Can you work these out from the drawing? Everything is in mm from the part's minimum corner. Give positions to 0.01 mm unless a question says otherwise; leave off trailing zeros. Write each loop counter-clockwise with the first axis right and the second up, starting at its lowest first coordinate (ties: lowest second). Pieces come first, ordered by that corner, then holes. Notation, with made-up numbers: (72, 1.5) - (87, 1.5) arc R23 ccw to (87, 38.5) - close; hole circle Ø1 at (-17.5, 23). An arc over 180 degrees is marked (long way). Return JSON: item names as keys, results as strings. Group by question number.
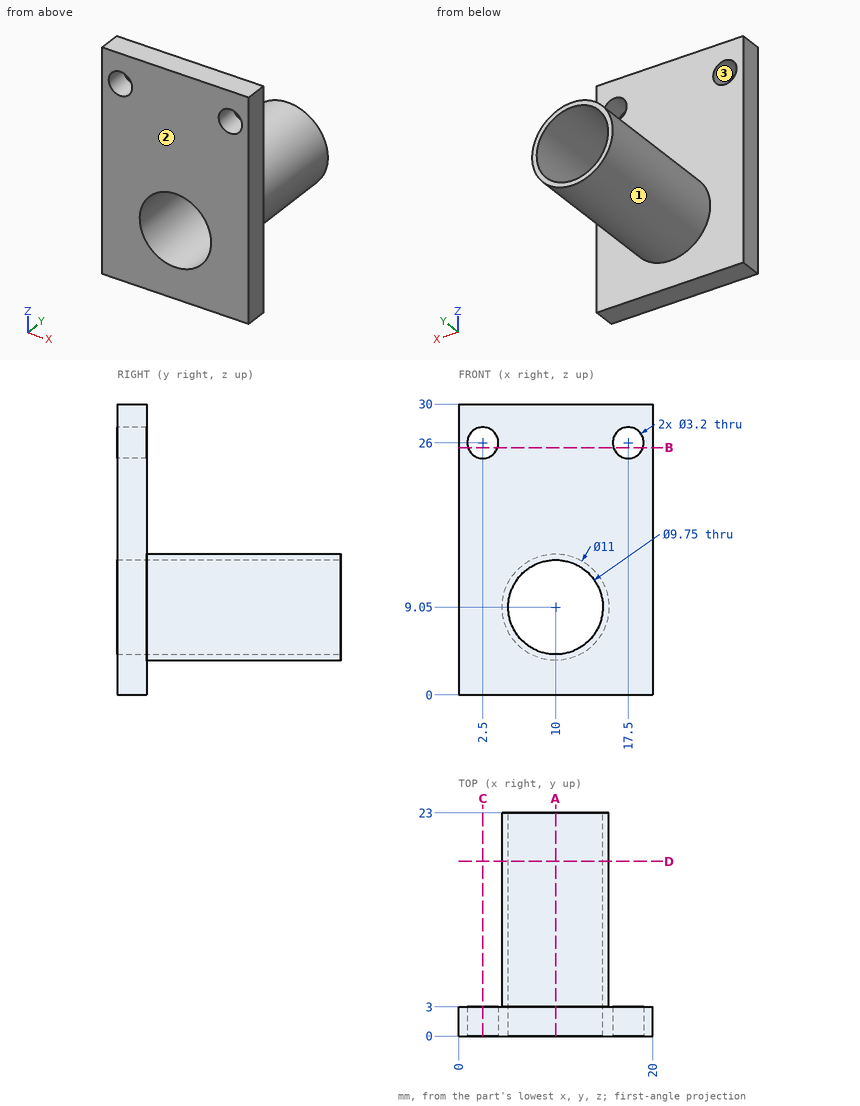
1) Will these pins go through, and if not, where does the flat tip stop? pin 1 Ø8 at (y, z) = (20, 20.5) entering from -X; pin 2 Ø6 at (x, y) = (11.5, 12.5) entering from +Z; pin 3 Ø4 at (x, z) = (11.5, 19.5) entering from +Y; pin 4 Ø2 at (y, z) = (5.5, 4.5) entering from +X.
2) Imagine slicing it at A-A, the plane x = 10. Write out the boundary of the cut face in (y, z) (3 decimals).
3) Imagine slicing it at B-B, the plane z = 25.5. Write out the boundary of the cut face in (x, y), and give its area (3 significant figures).
4) Imagine slicing it at D-D, the plane y = 18. Write out the boundary of the cut face in (x, z) (3 decimals).
5) Imagine slicing it at C-C, the plane x = 2.5. Write out the boundary of the cut face in (y, z).
6) We'd pull the mould along X, two halves only. Please class the marked faces 1, 2 and 3: pulls with the +X half, pulls with the -X half, needs draft (parallel to the pull), parting line crosses it, or undercut.
7) I need wall thicknesses on line 1 along X through (y, z) = (0.7, 26); line 2 along X through (y, z) = (5.75, 9.05) (3 decimals); line 3 along Y through (x, z) = (5, 1.5). Which ranges of each line are inside material? Lowest first, please.
Resolved:
{
 "1": {"pin 1": "through", "pin 2": "z = 14.55", "pin 3": "y = 3", "pin 4": "x = 14.2"},
 "2": {"outline": "(0, 0) - (3, 0) - (3, 3.55) - (23, 3.55) - (23, 4.175) - (0, 4.175) - close; (0, 13.925) - (23, 13.925) - (23, 14.55) - (3, 14.55) - (3, 30) - (0, 30) - close"},
 "3": {"outline": "(0, 0) - (0.98, 0) - (0.98, 3) - (0, 3) - close; (4.02, 0) - (15.98, 0) - (15.98, 3) - (4.02, 3) - close; (19.02, 0) - (20, 0) - (20, 3) - (19.02, 3) - close", "area": "41.8 mm^2"},
 "4": {"outline": "circle Ø11 at (10, 9.05); hole circle Ø9.75 at (10, 9.05)"},
 "5": {"outline": "(0, 0) - (3, 0) - (3, 24.4) - (0, 24.4) - close; (0, 27.6) - (3, 27.6) - (3, 30) - (0, 30) - close"},
 "6": {"face 1": "parting line crosses it", "face 2": "needs draft", "face 3": "undercut"},
 "7": {"line 1": "0 to 0.9, 4.1 to 15.9, 19.1 to 20", "line 2": "4.5 to 5.125, 14.875 to 15.5", "line 3": "0 to 3"}
}
